Here's how the part is built. I have some questions about the finished solid (model axes, mm). A direction names the side the tool comes from. Give positions to 0.01 mm unless a question says otherwise; leave off trailing zeros. Write each loop counter-clockwise with the first axis right and the second up, starting at its lowest first coordinate (ties: lowest second). Pieces come first, ordered by that corner, then holes. Notation, with made-up numbers: (20, 15) -> (27, 15) arc R38 ccw to (27, 54) -> close; hole circle Ø9 at (89.25, 77.25). An arc over 180 degrees is marked (long way). Return JSON: item names as keys, results as strings.
from build123d import *

# Parameters (mm, degrees)
BOSS_EXTRUDE1_DEPTH = 8.5
SKETCH2_W           = 17
SKETCH2_H           = 13
CUT_EXTRUDE1_DEPTH  = 17
CUT_EXTRUDE2_REACH  = 5
CUT_EXTRUDE3_DEPTH  = 4
SKETCH6_W           = 1
SKETCH6_H           = 1.85
SKETCH6_W_2         = 1.85
SKETCH6_H_2         = 1
BOSS_EXTRUDE2_DEPTH = 2


with BuildPart() as part:
    # Sketch1 → Boss-Extrude1 (new body, symmetric)
    with BuildSketch(Plane.XY):
        Polygon((0, 20), (0, 0), (20, 0), (20, 3), (3, 20), align=None)
    extrude(amount=BOSS_EXTRUDE1_DEPTH, both=True)

    # Sketch2 → Cut-Extrude1 (cut)
    with BuildSketch(Plane(origin=(0, 20, 0), x_dir=(1, 0, 0), z_dir=(0, 1, 0))):
        with Locations((11.5, 0)):
            Rectangle(SKETCH2_W, SKETCH2_H)
    extrude(amount=-CUT_EXTRUDE1_DEPTH, mode=Mode.SUBTRACT)

    # Sketch3 → Cut-Extrude2 (cut, up to next)
    with BuildSketch(Plane(origin=(3, 0, 0), x_dir=(0, 0, -1), z_dir=(1, 0, 0)), mode=Mode.PRIVATE) as cut_extrude2_sk1:
        with BuildLine():
            Line((-2.9, 8.5), (-2.9, 11.5))
            ThreePointArc((-2.9, 11.5), (0, 14.4), (2.9, 11.5))
            Line((2.9, 11.5), (2.9, 8.5))
            ThreePointArc((2.9, 8.5), (0, 5.6), (-2.9, 8.5))
        make_face()
    cut_extrude2_tool1 = extrude(cut_extrude2_sk1.sketch, amount=-CUT_EXTRUDE2_REACH, mode=Mode.PRIVATE) & part.part
    add(cut_extrude2_tool1.solids().sort_by_distance((3, 10, 0))[0], mode=Mode.SUBTRACT)

    # Sketch5 → Cut-Extrude3 (cut, through all)
    with BuildSketch(Plane(origin=(0, 3, 0), x_dir=(1, 0, 0), z_dir=(0, 1, 0))):
        with BuildLine():
            Line((11.5, -2.9), (8.5, -2.9))
            ThreePointArc((8.5, -2.9), (5.6, 0), (8.5, 2.9))
            Line((8.5, 2.9), (11.5, 2.9))
            ThreePointArc((11.5, 2.9), (14.4, 0), (11.5, -2.9))
        make_face()
    extrude(amount=-CUT_EXTRUDE3_DEPTH, mode=Mode.SUBTRACT)

    # Sketch6 → Boss-Extrude2 (add, symmetric)
    with BuildSketch(Plane.XY):
        with Locations((-0.5, 17.575)):
            Rectangle(SKETCH6_W, SKETCH6_H)
        with Locations((-0.5, 2.425)):
            Rectangle(SKETCH6_W, SKETCH6_H)
        with Locations((2.425, -0.5)):
            Rectangle(SKETCH6_W_2, SKETCH6_H_2)
        with Locations((17.575, -0.5)):
            Rectangle(SKETCH6_W_2, SKETCH6_H_2)
    extrude(amount=BOSS_EXTRUDE2_DEPTH, both=True)


solid = part.part
1. If we mould it in two halves opening along X, with no side actions, what happens to faces 1 (the face through (3, 14, 3)), 2 (the face through (3.35, -0.5, 0)), 3 (the face through (1.5, -0.5, 0)), 4 (the face through (8, 8, -8.5))? For each: released by +X, released by -X, zero draft, split by the parting line, or undercut.
Taken from the geometry:
{"face 1": "released by +X", "face 2": "undercut", "face 3": "released by -X", "face 4": "zero draft"}
2. Suppose I cut it at C-C, the plane x = 1. List the corners of the cut face in (y, z) for me, and give its area (3 significant figures).
Taken from the geometry:
{"outline": "(0, -8.5) -> (20, -8.5) -> (20, 8.5) -> (0, 8.5) -> close; hole (8.5, -2.9) -> (11.5, -2.9) arc R2.9 ccw to (11.5, 2.9) -> (8.5, 2.9) arc R2.9 ccw to start", "area": "296 mm²"}
3. For pin 1 Ø0.8 at (x, y) = (-0.5, 17.5) entering from -Z; pin 2 Ø1.1 at (y, z) = (-0.5, 1) entering from -X; pin 3 Ø1 at (x, z) = (13.5, 6.5) entering from -Y, each with a flat end and sliding along its axis, tell me the tip position at first contact or that it passes through.
Taken from the geometry:
{"pin 1": "stops at z = -2", "pin 2": "stops at x = 0", "pin 3": "stops at y = 0"}
4. Suppose I cut it at B-B, the plane y = 2. List the corners of the cut face in (x, z) for me, and give its area (3 significant figures).
Taken from the geometry:
{"outline": "(-1, -2) -> (0, -2) -> (0, -8.5) -> (20, -8.5) -> (20, 8.5) -> (0, 8.5) -> (0, 2) -> (-1, 2) -> close; hole (8.5, -2.9) -> (11.5, -2.9) arc R2.9 ccw to (11.5, 2.9) -> (8.5, 2.9) arc R2.9 ccw to start", "area": "300 mm²"}
5. Suppose I cut it at D-D, the plane z = 0. Count the separate pieces of the cut face and the enclosed holes in it, and give its area (3 significant figures).
Taken from the geometry:
{"separate pieces": "3", "enclosed holes": "0", "area": "65.6 mm²"}
6. Suppose I cut it at A-A, the plane x = 10. List the corners of the cut face in (y, z) for me, and give its area (3 significant figures).
Taken from the geometry:
{"outline": "(0, -8.5) -> (13, -8.5) -> (13, -6.5) -> (3, -6.5) -> (3, -2.9) -> (0, -2.9) -> close; (0, 2.9) -> (3, 2.9) -> (3, 6.5) -> (13, 6.5) -> (13, 8.5) -> (0, 8.5) -> close", "area": "73.6 mm²"}
7. If I drill on line 1 (Z direction, x = 11.5, y = 7.75); line 2 (Z direction, x = 2.25, y = 9.25); line 3 (Y direction, x = 3.25, z = 2.5), over which ranges is the centre line in solid material (lowest first)? Write a range as [from, to].
Taken from the geometry:
{"line 1": "z = [-8.5, -6.5], [6.5, 8.5]", "line 2": "z = [-8.5, -2.9], [2.9, 8.5]", "line 3": "y = [0, 3]"}
8. Which directions (+Z, -Z, +X, -X, +Y, -Y) give clear straight access to the entire face, cutting with the end or side of a thin tool? Please do faces 5 (the face through (-0.5, 2.4, -2)), 6 (the face through (-0.5, 1.5, 0)), 7 (the face through (13, 3, -3)).
Taken from the geometry:
{"face 5": "-Z, -X, +Y, -Y", "face 6": "+Z, -Z, -X, -Y", "face 7": "+X, +Y"}
